Source: CAD feature listing. Evaluate the final solid. Frame: model axes, mm. Give positions to 0.01 mm unless a question says otherwise; leave off trailing zeros. Loops run counter-clockwise (first coordinate to the right, second up) from the corner with the lowest first, then second, coordinate; pieces in that order, holes last. Notation, with made-up numbers: M -16,64 L 37,64 A16 ccw 37,93 Z; hole C 52.25,-27.75 d7. An arc over 180 degrees is marked long. Answer in a Markdown table with one row per item.
```python
from build123d import *

# Parameters (mm, degrees)
BOX023_W     = 19
BOX023_H     = 1400
BOX023_DEPTH = 190
BOX024_W     = 19
BOX024_H     = 1438
BOX024_DEPTH = 460
BOX021_W     = 19
BOX021_H     = 925
BOX021_DEPTH = 120


with BuildPart() as cube023:
    # Box023 → Box023 (new body)
    with BuildSketch(Plane(origin=(2019, 281, 950), x_dir=(1, 0, 0), z_dir=(0, 0, 1))):
        with Locations((9.5, 700)):
            Rectangle(BOX023_W, BOX023_H)
    extrude(amount=BOX023_DEPTH)


with BuildPart() as cube024:
    # Box024 → Box024 (new body)
    with BuildSketch(Plane(origin=(2019, 262, 1140), x_dir=(1, 0, 0), z_dir=(0, 0, 1))):
        with Locations((9.5, 719)):
            Rectangle(BOX024_W, BOX024_H)
    extrude(amount=BOX024_DEPTH)


with BuildPart() as headboard:
    # Box021 → Box021 (new body)
    with BuildSketch(Plane(origin=(2019, 575, 830), x_dir=(1, 0, 0), z_dir=(0, 0, 1))):
        with Locations((9.5, 462.5)):
            Rectangle(BOX021_W, BOX021_H)
    extrude(amount=BOX021_DEPTH)

    # Fusion: union Cube023, Cube024
    add(cube023.part)
    add(cube024.part)


solid = headboard.part
```
Q1. Ray query, probe 1 along Z at (x, y) = (2035.25, 1614.5); probe 2 along Y at (x, z) = (2020.75, 1009); probe 3 along Y at (x, z) = (2024, 898.5). Return the intervals inside material, ascending. Write a range as from..to.
Values follow:
| item | result |
|---|---|
| probe 1 | 950..1600 |
| probe 2 | 281..1681 |
| probe 3 | 575..1500 |
Q2. Section query C-C (y = 477). Output: boundary loops of the cut face in (x, z), plus the area to 4 significant figures.
Values follow:
| item | result |
|---|---|
| outline | M 2019,950 L 2038,950 L 2038,1600 L 2019,1600 Z |
| area | 12,350 mm^2 |
Q3. Section query B-B (z = 917.5). Output: boundary loops of the cut face in (x, y).
Values follow:
| item | result |
|---|---|
| outline | M 2019,575 L 2038,575 L 2038,1500 L 2019,1500 Z |
Q4. Section query A-A (x = 2034.5). Output: boundary loops of the cut face in (y, z), plus the area to 3 significant figures.
Values follow:
| item | result |
|---|---|
| outline | M 262,1140 L 281,1140 L 281,950 L 575,950 L 575,830 L 1500,830 L 1500,950 L 1681,950 L 1681,1140 L 1700,1140 L 1700,1600 L 262,1600 Z |
| area | 1,040,000 mm^2 |
Q5. Contact query for flat-ended pins moving along their axis: pin 1 Ø9.5 at (x, z) = (2032, 890.5) entering from -Y; pin 2 Ø3 at (x, z) = (2029, 1092) entering from -Y; pin 3 Ø9.5 at (x, y) = (2027.5, 469.5) entering from -Z. Output: stop coordinate, or through.
Values follow:
| item | result |
|---|---|
| pin 1 | y = 575 |
| pin 2 | y = 281 |
| pin 3 | z = 950 |
